from build123d import *

# Parameters (mm, degrees)
SKETCH1_R           = 5
BOSS_EXTRUDE1_DEPTH = 20
BOSS_EXTRUDE2_DEPTH = 2
SKETCH3_R           = 2
CUT_EXTRUDE1_DEPTH  = 23
BOSS_EXTRUDE3_DEPTH = 5
SKETCH5_W           = 2
SKETCH5_H           = 27.667167525
BOSS_EXTRUDE4_DEPTH = 5
SKETCH6_R           = 3.75
BOSS_EXTRUDE5_DEPTH = 2.5
SKETCH7_R           = 1.5
BOSS_EXTRUDE6_DEPTH = 20


with BuildPart() as part:
    # Sketch1 → Boss-Extrude1 (new body)
    with BuildSketch(Plane(origin=(0, 0, 0), x_dir=(0, 0, -1), z_dir=(1, 0, 0))):
        Circle(SKETCH1_R)
    extrude(amount=BOSS_EXTRUDE1_DEPTH)

    # Sketch2 → Boss-Extrude2 (add)
    with BuildSketch(Plane(origin=(20, 0, 0), x_dir=(0, 0, -1), z_dir=(1, 0, 0))):
        with BuildLine():
            Line((-5, 0), (-5, -17.185208198))
            Line((-5, -17.185208198), (5, -17.185208198))
            Line((5, -17.185208198), (5, 0))
            ThreePointArc((5, 0), (0, 5), (-5, 0))
        make_face()
    extrude(amount=BOSS_EXTRUDE2_DEPTH)

    # Sketch3 → Cut-Extrude1 (cut, through all)
    with BuildSketch(Plane(origin=(22, 0, 0), x_dir=(0, 0, -1), z_dir=(1, 0, 0))):
        Circle(SKETCH3_R)
    extrude(amount=-CUT_EXTRUDE1_DEPTH, mode=Mode.SUBTRACT)

    # Sketch4 → Boss-Extrude3 (add, symmetric)
    with BuildSketch(Plane.XY):
        Polygon((20, -17.185208198), (33.506911319, -33.834240512), (35.506911319, -33.834240512), (22, -17.185208198), align=None)
    extrude(amount=BOSS_EXTRUDE3_DEPTH, both=True)

    # Sketch5 → Boss-Extrude4 (add, symmetric)
    with BuildSketch(Plane.XY):
        with Locations((34.506911319, -47.667824275)):
            Rectangle(SKETCH5_W, SKETCH5_H)
    extrude(amount=BOSS_EXTRUDE4_DEPTH, both=True)

    # Sketch6 → Boss-Extrude5 (add)
    with BuildSketch(Plane(origin=(35.506911319, 0, 0), x_dir=(0, 0, -1), z_dir=(1, 0, 0))):
        with Locations((0, -54.001408037)):
            Circle(SKETCH6_R)
    extrude(amount=BOSS_EXTRUDE5_DEPTH)

    # Sketch7 → Boss-Extrude6 (add)
    with BuildSketch(Plane(origin=(38.006911319, 0, 0), x_dir=(0, 0, -1), z_dir=(1, 0, 0))):
        with Locations((0, -54.001408037)):
            Circle(SKETCH7_R)
    extrude(amount=BOSS_EXTRUDE6_DEPTH)


solid = part.part
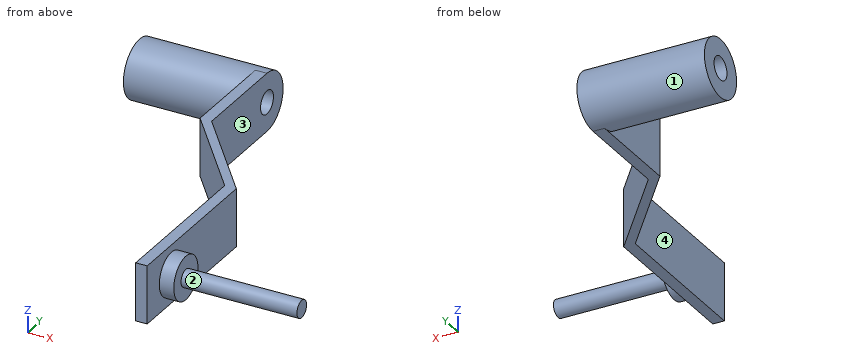
For this review, take the finished solid that the model builds, in its own axes (mm). Face numbers are marked on the shaded views. A direction names the side the tool comes from. Round coordinates to 2 decimals unless told otherwise and drop trailing zeros. Write each loop counter-clockwise with the first axis right and the second up, starting at its lowest first coordinate (ties: lowest second). Pieces come first, ordered by that corner, then holes. Notation, with made-up numbers: (33.25, 84) - (38.25, 84) arc R21 ccw to (38.25, 92) - close; hole circle Ø6 at (43.5, -21). An arc over 180 degrees is marked (long way). Use a Markdown table: item, result.
Q1. Wall thickness on line 1 along Y through (x, z) = (13, 0); line 2 along X through (y, z) = (-10.5, 0.75); line 3 along X through (y, z) = (1, -4): over which ranges is each line inside the solid? List them lowest first.
Derived:
| item | result |
|---|---|
| line 1 | y = -5 to -2, 2 to 5 |
| line 2 | x = 20 to 22 |
| line 3 | x = 0 to 22 |
Q2. We need section B-B (x = 14). Give the boundary of the cut face in (y, z).
Derived:
| item | result |
|---|---|
| outline | circle Ø10 at (0, 0); hole circle Ø4 at (0, 0) |
Q3. We need section C-C (y = -13.5). Give the boundary of the cut face in (x, z), plus the area to 3 significant figures.
Derived:
| item | result |
|---|---|
| outline | (20, -5) - (22, -5) - (22, 5) - (20, 5) - close |
| area | 20.0 mm2 |
Q4. Machinability: for the marked faces 1, 2, 3 and 4, which of the approach directions +Z, -Z, +X, -X, +Y, -Y give a long, thin tool a straight path to every point of the face, cutting with its end or side? Answer none if there is none.
Derived:
| item | result |
|---|---|
| face 1 | -X |
| face 2 | +X |
| face 3 | +Z, -Z, +X, +Y |
| face 4 | +Z, -Z, -X, -Y |
Q5. We need section D-D (x = 40). Give the boundary of the cut face in (y, z).
Derived:
| item | result |
|---|---|
| outline | circle Ø3 at (-54, 0) |
Q6. Clearance check with flat-ended pins moving along their axes: pin 1 (1 mm diameter, centred on y = -53, z = 0, fed in from -X); pin 2 (5 mm diameter, centred on y = -10.5, z = -2, fed in from +X); pin 3 (5 mm diameter, centred on y = -8.5, z = -2, fed in from -X). State where each tip first meets the part, or that it passes through.
Derived:
| item | result |
|---|---|
| pin 1 | stops at x = 33.51 |
| pin 2 | stops at x = 22 |
| pin 3 | stops at x = 20 |
Q7. We need section A-A (z = 0). Give the boundary of the cut face in (x, y).
Derived:
| item | result |
|---|---|
| outline | (0, -5) - (20, -5) - (20, -17.19) - (33.51, -33.83) - (33.51, -61.5) - (35.51, -61.5) - (35.51, -57.75) - (38.01, -57.75) - (38.01, -55.5) - (58.01, -55.5) - (58.01, -52.5) - (38.01, -52.5) - (38.01, -50.25) - (35.51, -50.25) - (35.51, -33.83) - (22, -17.19) - (22, -2) - (0, -2) - close; (0, 2) - (22, 2) - (22, 5) - (0, 5) - close |
